```python
from build123d import *

# Parameters (mm, degrees)
CHAMFER_1_SIZE           = 2
CHAMFER_1_SIZE2          = 3.464101615
CHAMFER_2_SIZE           = 1.5
SKETCH_2_W               = 2
SKETCH_2_H               = 31
CUT_EXTRUDE_1_DEPTH      = 32.559467676
PATTERN_CIRCULAR_1_COUNT = 10


with BuildPart() as part:
    # 草图1 → 旋转1 (revolve)
    with BuildSketch(Plane.XY, mode=Mode.PRIVATE) as revolve_1_sk:
        Polygon((-2.5, 0), (-2.5, 8), (-4.75, 8), (-4.75, 12), (-14.5, 12), (-14.5, 26), (-20, 26), (-20, 20.3), (-17, 20.3), (-17, 6), (-6.5, 6), (-6.5, 5), (-4.5, 5), (-4.5, 0), align=None)
    revolve(revolve_1_sk.sketch.rotate(Axis((0, 0, 0), (0, 1, 0)), 270), axis=Axis((0, 0, 0), (0, 1, 0)))

    # 倒角1
    chamfer_1_edges = [part.edges().sort_by_distance(p)[0] for p in [
        (0, 26, 14.5),
    ]]
    chamfer_1_side = [part.faces().sort_by_distance(p)[0] for p in [
        (0, 19, 14.5),
    ]]
    chamfer(chamfer_1_edges, length=CHAMFER_1_SIZE, length2=CHAMFER_1_SIZE2, reference=chamfer_1_side[0])

    # 倒角2
    chamfer_2_edges = [part.edges().sort_by_distance(p)[0] for p in [
        (0, 26, 20),
    ]]
    chamfer(chamfer_2_edges, length=CHAMFER_2_SIZE)

    # 草图2 → 切除-拉伸1 (cut, through all)
    with BuildSketch(Plane(origin=(0, 12, 0), x_dir=(1, 0, 0), z_dir=(0, 1, 0))):
        Rectangle(SKETCH_2_W, SKETCH_2_H)
    cut_extrude_1 = extrude(amount=CUT_EXTRUDE_1_DEPTH, mode=Mode.SUBTRACT)

    # 阵列(圆周)1: 切除-拉伸1 ×10 about axis
    pattern_circular_1_axis = Axis((0, 0, 0), (0, 1, 0))
    for i in range(1, PATTERN_CIRCULAR_1_COUNT):
        add(cut_extrude_1.rotate(pattern_circular_1_axis, i * 360 / PATTERN_CIRCULAR_1_COUNT), mode=Mode.SUBTRACT)


solid = part.part
```
Check sheet for the modelled part. Datum: model origin and axes. Units: mm. A direction names the side the tool comes from. Coordinates: 2 decimals unless noted, no trailing zeros. Order: outer loops, then holes, each group sorted by start corner. A loop starts at its lowest first (then second) coordinate and runs counter-clockwise, first axis right, second up. Notation, with made-up numbers: M 27.5,-28 L 53.5,-28 A13 cw 53.5,-9 Z; hole C 13.5,-32 d4. An arc over 180 degrees is marked long. Write each question's results on one line, items separated by ' | '. Start each with the question number.
1. Mould release check, pull along Z, two halves, no side actions. Record for faces 4 (the face through (-4, 12, 3)), 5 (the face through (15, 20.3, 9)), 6 (the face through (-1.352, 2.465, -4.292)): +Z half, -Z half, draft (parallel to the pull), parting line (faces both ways), or undercut.
2. Go/stop test with flat-tipped pins: P1, Ø5, axis at x = -3, z = 15, coming from the +Y side; P2, Ø3, axis at y = 9, z = -6.5, coming from the -X side; P3, Ø8, axis at x = -8, y = 8.5, coming from the -Z side; P4, Ø4.5, axis at x = 0, z = 0, coming from the +Y side. Record where each tip stops, or that it passes through.
3. Cross-section at D-D on y = 2.5. Record the cut outline in (x, z).
4. Access from +Z, -Z, +X, -X, +Y, -Y to the whole of each face (thin tool, end or side, straight path). Record for faces 1 (the face through (2, 0, -2)), 2 (the face through (3.955, 5.493, 5.158)), 3 (the face through (-13.934, 18.21, 5.579)).
5. Cross-section at C-C on y = 11.25. Record the cut outline in (x, z), and give its area (3 significant figures).
6. Material ranges on probe 1 along X at (y, z) = (6.5, 0); probe 2 along X at (y, z) = (9.6, 0); probe 3 along Z at (x, y) = (12.5, 13), recorded low to high.
Checks:
1) face 4: undercut | face 5: draft | face 6: parting line
2) P1: stops at y = 25.9 | P2: stops at x = -16.25 | P3: stops at z = -16.52 | P4: passes through
3) outline: C 0,0 d9; hole C 0,0 d5
4) face 1: +Z, -Z, +X, -X, -Y | face 2: -Y | face 3: +Y
5) outline: C 0,0 d34; hole C 0,0 d9.5 | area: 837 mm²
6) probe 1: x = -17 to -2.5, 2.5 to 17 | probe 2: x = -17 to -4.75, 4.75 to 17 | probe 3: z = -11.52 to -7.35, 7.35 to 11.52
